from build123d import *

# Parameters (mm, degrees)
F1_DEPTH = 100


with BuildPart() as f1:
    # F0 (on Right) → F1 (new body)
    with BuildSketch(Plane.YZ):
        Polygon((6.5, 6.5), (0, 0), (0, -20), (100, -20), (100, 0), (80, 0), (80, -1.5), (76.5, -1.5), (76.5, 0), (72, 4.5), (70, 4.5), (65.5, 0), (65.5, -15), (39.5, -15), (39.5, 0), (22.5, 0), (22.5, -1.5), (16, -1.5), (16, 0), (9.5, 6.5), align=None)
    extrude(amount=F1_DEPTH)


solid = f1.part
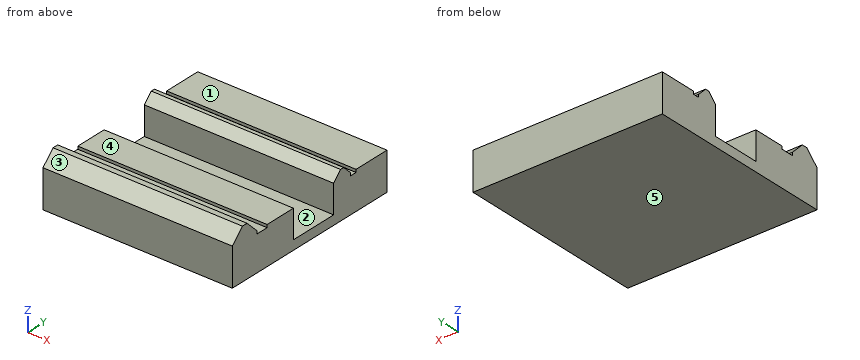
Geometry: final body of the model. Coordinates: model frame, mm. Face numbers are marked on the shaded views. A direction names the side the tool comes from. Coordinates: 2 decimals unless noted, no trailing zeros. Loops run counter-clockwise (first coordinate to the right, second up) from the corner with the lowest first, then second, coordinate; pieces in that order, holes last. Notation, with made-up numbers: (72.5, 86) - (78.5, 86) arc R14 ccw to (78.5, 103) - close; hole circle Ø9 at (-32.75, 45). An arc over 180 degrees is marked (long way). One line per question, with ' | ' between items. Start each with the question number.
(1) Cut plane C-C on z = 1.5. Output: boundary loops of the cut face in (x, y).
(2) Cut plane A-A on z = -8.25. Output: boundary loops of the cut face in (x, y), and give its area (3 significant figures).
(3) First-contact query: pin 1 (6 mm diameter, centred on x = 76, y = 84.5, fed in from +Z); pin 2 (1 mm diameter, centred on x = 34.5, y = 71, fed in from +Z); pin 3 (1 mm diameter, centred on x = 70, y = 78, fed in from +Z). Flat tips, straight axial feed; report the tip coordinate or a pass-through.
(4) Ray query, L1, parallel to Y at x = 75, z = -1; L2, parallel to Y at x = 20.5, z = -4; L3, parallel to Z at x = 23, y = 56.5. Return the intervals inside material, ascending. Write a range as from..to.
(5) Reachability of the marked faces 4 and 5 from +Z, -Z, +X, -X, +Y, -Y: full face, straight path, thin tool, end or side. Return the list, or none.
(6) Draft query along Y for the marked faces 1, 2 and 3. Return one class per face: +Y half, -Y half, draft (parallel to the pull), parting line (faces both ways), or undercut.
(7) Cut plane B-B on x = 48. Output: boundary loops of the cut face in (y, z).
(8) Cut plane D-D on y = 29.5. Output: boundary loops of the cut face in (x, z), and give its area (3 significant figures).
Here are the results:
1) outline: (0, 1.5) - (100, 1.5) - (100, 14.5) - (0, 14.5) - close; (0, 67) - (100, 67) - (100, 75) - (0, 75) - close
2) outline: (0, 0) - (100, 0) - (100, 39.5) - (0, 39.5) - close; (0, 65.5) - (100, 65.5) - (100, 100) - (0, 100) - close | area: 7,400 mm²
3) pin 1: z = 0 | pin 2: z = 4.5 | pin 3: z = -1.5
4) L1: 0..16, 22.5..39.5, 65.5..76.5, 80..100 | L2: 0..39.5, 65.5..100 | L3: -20..-15
5) face 4: +Z, +X, -X | face 5: -Z, +X, -X, +Y, -Y
6) face 1: draft | face 2: undercut | face 3: -Y half
7) outline: (0, -20) - (100, -20) - (100, 0) - (80, 0) - (80, -1.5) - (76.5, -1.5) - (76.5, 0) - (72, 4.5) - (70, 4.5) - (65.5, 0) - (65.5, -15) - (39.5, -15) - (39.5, 0) - (22.5, 0) - (22.5, -1.5) - (16, -1.5) - (16, 0) - (9.5, 6.5) - (6.5, 6.5) - (0, 0) - close
8) outline: (0, -20) - (100, -20) - (100, 0) - (0, 0) - close | area: 2,000 mm²
